from build123d import *

# Parameters (mm, degrees)
SKETCH1_R                = 130
SKETCH1_R_2              = 11.1125
BOSS_EXTRUDE1_DEPTH      = 87.5
SKETCH2_R                = 100
CUT_EXTRUDE1_DEPTH       = 10
CUT_EXTRUDE2_START       = -166
SKETCH3_R                = 6
CUT_EXTRUDE2_DEPTH       = 177
CIRPATTERN1_COUNT        = 5
SKETCH4_R                = 30.2387
SKETCH4_R_2              = 11.1125
BOSS_EXTRUDE2_DEPTH      = 2
BOSS_EXTRUDE2_DEPTH_BACK = 7


with BuildPart() as part:
    # Sketch1 → Boss-Extrude1 (new body, symmetric)
    with BuildSketch(Plane.XY):
        Circle(SKETCH1_R)
        Circle(SKETCH1_R_2, mode=Mode.SUBTRACT)
    extrude(amount=BOSS_EXTRUDE1_DEPTH, both=True)

    # Sketch2 → Cut-Extrude1 (cut)
    with BuildSketch(Plane.XY.offset(87.5)):
        Circle(SKETCH2_R)
    cut_extrude1 = extrude(amount=-CUT_EXTRUDE1_DEPTH, mode=Mode.SUBTRACT)

    # Mirror1: Cut-Extrude1 across plane
    add(cut_extrude1.mirror(Plane.XY), mode=Mode.SUBTRACT)

    # Sketch3 → Cut-Extrude2 (cut)
    with BuildSketch(Plane.XY.offset(77.5).offset(CUT_EXTRUDE2_START)):
        with Locations((0, 75)):
            Circle(SKETCH3_R)
    cut_extrude2 = extrude(amount=CUT_EXTRUDE2_DEPTH, mode=Mode.SUBTRACT)

    # CirPattern1: Cut-Extrude2 ×5 about axis
    cirpattern1_axis = Axis((0, 0, 0), (0, 0, 1))
    for i in range(1, CIRPATTERN1_COUNT):
        add(cut_extrude2.rotate(cirpattern1_axis, i * 360 / CIRPATTERN1_COUNT), mode=Mode.SUBTRACT)

    # Sketch4 → Boss-Extrude2 (add, two sides)
    with BuildSketch(Plane.XY.offset(77.5)) as boss_extrude2_sk:
        Circle(SKETCH4_R)
        Circle(SKETCH4_R_2, mode=Mode.SUBTRACT)
    extrude(amount=BOSS_EXTRUDE2_DEPTH)
    extrude(boss_extrude2_sk.sketch, amount=-BOSS_EXTRUDE2_DEPTH_BACK)

    # Sketch5 → Cut-Revolve1 (revolve, cut)
    with BuildSketch(Plane(origin=(0, 0, 0), x_dir=(1, 0, 0), z_dir=(0, 1, 0))):
        Polygon((130, 84.5), (124, 81.035898385), (124, -81.035898385), (130, -84.5), align=None)
    revolve(axis=Axis((0, 0, 0), (0, 0, -1)), mode=Mode.SUBTRACT)


solid = part.part
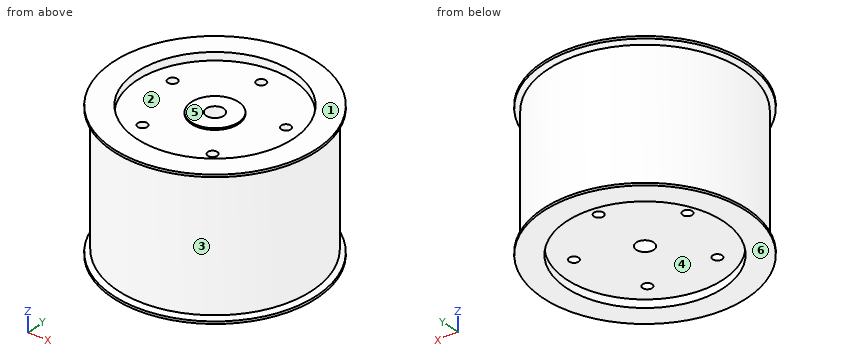
Verification items for the finished model (mm, model axes). Face numbers are marked on the shaded views. A direction names the side the tool comes from. Coordinates: 2 decimals unless noted, no trailing zeros. Write each loop counter-clockwise with the first axis right and the second up, starting at its lowest first coordinate (ties: lowest second). Pieces come first, ordered by that corner, then holes. Notation, with made-up numbers: (-3, 84.25) -> (26, 84.25) arc R18 cw to (26, 105.25) -> close; hole circle Ø4 at (48, 46.25). An arc over 180 degrees is marked (long way). One line per item, written item: value. Start each with the question number.
Q1. Access from +Z, -Z, +X, -X, +Y, -Y to the whole of each face (thin tool, end or side, straight path). Record for the marked faces 4, 5 and 6.
Q2. Mould release check, pull along Y, two halves, no side actions. Record for the marked faces 1, 2 and 3: pulls with the +Y half, pulls with the -Y half, needs draft (parallel to the pull), parting line crosses it, or undercut.
Q3. Thickness scan on L1, parallel to Y at x = 0, z = 8; L2, parallel to X at y = -3, z = 66; L3, parallel to Z at x = 16.5, y = -64.5. Record the ranges inside material, lowest first. Write a range as from..to.
Q4. Go/stop test with flat-tipped pins: P1, Ø14, axis at x = 71.33, y = 23.18, coming from the -Z side; P2, Ø1.5, axis at x = -10, z = 2.5, coming from the +Y side; P3, Ø10, axis at x = -46.5, z = -39, coming from the -Y side. Record where each tip stops, or that it passes through.
Q5. Cross-section at A-A on y = 0. Enter the section's corners in (x, z), and give its area (3 significant figures).
Q6. Cross-section at B-B on x = 0. State how many separate pieces and enclosed holes the cut face has, and give its area (3 significant figures).
Q7. Cross-section at C-C on z = -2. Enter the section's corners in (x, y) (1 decimal).
Checked values:
1. face 4: -Z
1. face 5: +Z
1. face 6: -Z, +X, -X, +Y, -Y
2. face 1: needs draft
2. face 2: undercut
2. face 3: parting line crosses it
3. L1: y = -124..-11.11, 11.11..69, 81..124
3. L2: x = -123.96..-10.7, 10.7..123.96
3. L3: z = -77.5..77.5
4. P1: stops at z = -77.5
4. P2: stops at y = 123.65
4. P3: stops at y = -116.85
5. outline: (-130, -87.5) -> (-100, -87.5) -> (-100, -77.5) -> (-11.11, -77.5) -> (-11.11, 79.5) -> (-30.24, 79.5) -> (-30.24, 77.5) -> (-100, 77.5) -> (-100, 87.5) -> (-130, 87.5) -> (-130, 84.5) -> (-124, 81.04) -> (-124, -81.04) -> (-130, -84.5) -> close; (11.11, -77.5) -> (100, -77.5) -> (100, -87.5) -> (130, -87.5) -> (130, -84.5) -> (124, -81.04) -> (124, 81.04) -> (130, 84.5) -> (130, 87.5) -> (100, 87.5) -> (100, 77.5) -> (30.24, 77.5) -> (30.24, 79.5) -> (11.11, 79.5) -> close
5. area: 36,100 mm²
6. separate pieces: 3
6. enclosed holes: 0
6. area: 34,300 mm²
7. outline: circle Ø248 at (0, 0); hole circle Ø12 at (-71.3, 23.2); hole circle Ø12 at (-44.1, -60.7); hole circle Ø22.2 at (0, 0); hole circle Ø12 at (0, 75); hole circle Ø12 at (44.1, -60.7); hole circle Ø12 at (71.3, 23.2)
